Could you check a few things on this model? Use its own coordinates, in mm. Face numbers are marked on the shaded views. A direction names the side the tool comes from. Round coordinates to 2 decimals unless told otherwise and drop trailing zeros. Loops run counter-clockwise (first coordinate to the right, second up) from the corner with the lowest first, then second, coordinate; pieces in that order, holes last. Notation, with made-up numbers: (80, 71.25) -> (109, 71.25) arc R14 cw to (109, 78.25) -> close; hole circle Ø10 at (42, 68). An arc over 180 degrees is marked (long way). One line per item, written item: value.
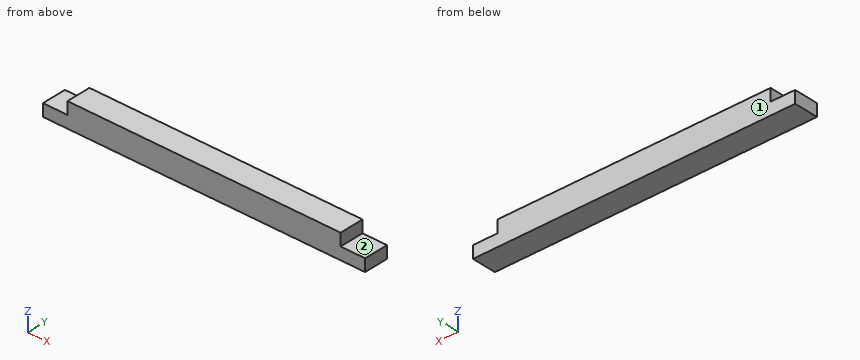
```python
from build123d import *

# Parameters (mm, degrees)
F0_W     = 88.9
F0_H     = 88.9
F1_DEPTH = 673.1
F2_W     = 88.9
F2_H     = 44.45
F3_DEPTH = 88.901
F4_W     = 88.9
F4_H     = 88.9
F5_DEPTH = 88.901


with BuildPart() as f1:
    # F0 (on Right) → F1 (new body, symmetric)
    with BuildSketch(Plane.YZ):
        Rectangle(F0_W, F0_H)
    extrude(amount=F1_DEPTH, both=True)

    # F2 (on face) → F3 (cut, through all)
    with BuildSketch(Plane.XZ.offset(44.45)):
        with Locations((-539.75, 22.225)):
            Rectangle(F2_W, F2_H)
        with Locations((539.75, 22.225)):
            Rectangle(F2_W, F2_H)
    extrude(amount=-F3_DEPTH, mode=Mode.SUBTRACT)

    # F4 (on face) → F5 (cut, through all)
    with BuildSketch(Plane.XZ.offset(44.45)):
        with Locations((-628.65, 0)):
            Rectangle(F4_W, F4_H)
        with Locations((628.65, 0)):
            Rectangle(F4_W, F4_H)
    extrude(amount=-F5_DEPTH, mode=Mode.SUBTRACT)


solid = f1.part
```
(1) For pin 1 Ø10 at (y, z) = (-19, 29.5) entering from +X; pin 2 Ø12 at (y, z) = (-30.5, 25.5) entering from -X, each with a flat end and sliding along its axis, tell me the tip position at first contact or that it passes through.
Results below:
pin 1: stops at x = 495.3
pin 2: stops at x = -495.3
(2) Imagine slicing it at B-B on z = 32.5. Write out the boundary of the cut face in (x, y).
Results below:
outline: (-495.3, -44.45) -> (495.3, -44.45) -> (495.3, 44.45) -> (-495.3, 44.45) -> close
(3) On a 3-axis mill with a long thin cutter (end or side, diameter ignored), from which of +Z, -Z, +X, -X, +Y, -Y can I reach the whole of each face in a straight line? I mean the marked faces 1 and 2. Say none if no direction works.
Results below:
face 1: +Z, -Z, +X, -X, +Y
face 2: +Z, +X, +Y, -Y
(4) Imagine slicing it at A-A on y = 17.5. Write out the boundary of the cut face in (x, z).
Results below:
outline: (-584.2, -44.45) -> (584.2, -44.45) -> (584.2, 0) -> (495.3, 0) -> (495.3, 44.45) -> (-495.3, 44.45) -> (-495.3, 0) -> (-584.2, 0) -> close
(5) Please list where these lines run through material, in increasing order: L1, parallel to X at y = 36.5, z = 31; L2, parallel to Z at x = 496.5, y = -30.
Results below:
L1: x = -495.3 to 495.3
L2: z = -44.45 to 0
